Input: part model. Units: mm. Frame: model coordinates. A direction names the side the tool comes from. Give positions to 0.01 mm unless a question says otherwise; leave off trailing zeros. Loops run counter-clockwise (first coordinate to the right, second up) from the corner with the lowest first, then second, coordinate; pieces in that order, holes last.
from build123d import *

# Parameters (mm, degrees)
F0_R     = 3.33375
F1_DEPTH = 4.7625
F2_R     = 2.38125
F3_DEPTH = 76.2
F4_R     = 3.33375
F5_DEPTH = 4.7625
F6_R     = 1.905


with BuildPart() as f1:
    # F0 (on Top) → F1 (new body)
    with BuildSketch(Plane.XY):
        Circle(F0_R)
    extrude(amount=F1_DEPTH)

    # F2 (on face) → F3 (join)
    with BuildSketch(Plane(origin=(0, 0, 0), x_dir=(1, 0, 0), z_dir=(0, 0, -1))):
        Circle(F2_R)
    extrude(amount=F3_DEPTH)

    # F4 (on face) → F5 (join)
    with BuildSketch(Plane(origin=(0, 0, -76.2), x_dir=(1, 0, 0), z_dir=(0, 0, -1))):
        Circle(F4_R)
    extrude(amount=F5_DEPTH)

    # F6
    f6_edges = [f1.edges().sort_by_distance(p)[0] for p in [
        (-3.33375, 0, 4.7625),
        (-3.33375, 0, -80.9625),
    ]]
    fillet(f6_edges, radius=F6_R)


solid = f1.part
(1) Ray query, probe 1 along Z at (x, y) = (1.5, 0.75); probe 2 along Z at (x, y) = (-1, 2.5); probe 3 along Z at (x, y) = (-3, -1). Return the intervals inside material, ascending.
Values follow:
probe 1: z = -80.95 to 4.75
probe 2: z = -80.48 to -76.2, 0 to 4.28
probe 3: z = -79.85 to -76.2, 0 to 3.65
(2) Reachability of faces 3 (the cylindrical face through (-0.434, -3.305, -77.609)), 4 (the flat face through (2.2, -1.4, 0)) from +Z, -Z, +X, -X, +Y, -Y: full face, straight path, thin tool, end or side. Return the list, or none.
Values follow:
face 3: +Z, -Z
face 4: none
(3) Pin query (flat end, axial travel): pin 1 Ø1 at (x, y) = (-2.5, 1.5) entering from -Z; pin 2 Ø1.5 at (x, y) = (0, 2.5) entering from +Z; pin 3 Ø1.5 at (y, z) = (-0.5, -30) entering from -X. Return the tip coordinate at first contact, or that it passes through.
Values follow:
pin 1: stops at z = -80.69
pin 2: stops at z = 4.74
pin 3: stops at x = -2.38
(4) Cut plane A-A (z = -59.5). Return the cut outline in (x, y), and give its area (3 significant figures).
Values follow:
outline: circle Ø4.76 at (0, 0)
area: 17.8 mm2
(5) Mould query, pull axis X, two halves, no side actions, for faces 1 (the flat face through (2.2, 1.4, -76.2)), 2 (the cylindrical face through (-0.434, 3.305, 1.409)). Classes: +X half, -X half, draft (parallel to the pull), parting line (faces both ways), or undercut.
Values follow:
face 1: draft
face 2: parting line
